Design review of the part built by this model. Coordinates are the model's own, in mm. Face numbers are marked on the shaded views. Coordinates: 2 decimals unless noted, no trailing zeros. Loops run counter-clockwise (first coordinate to the right, second up) from the corner with the lowest first, then second, coordinate; pieces in that order, holes last. Notation, with made-up numbers: (-16.5, 30) -> (8.5, 30) arc R13 cw to (8.5, 43) -> close; hole circle Ø9 at (49, 89). An arc over 180 degrees is marked (long way). Answer as a JSON object with one key per item and string values.
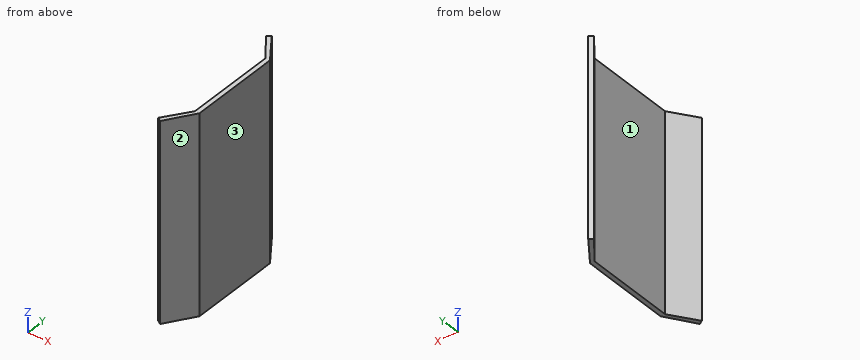
```python
from build123d import *

# Parameters (mm, degrees)
F0_W     = 30
F0_H     = 600
F1_DEPTH = 1300


with BuildPart() as f1:
    # F0 (on Top) → F1 (new body)
    with BuildSketch(Plane.XY):
        with Locations((-14.494546, -122.679873)):
            Rectangle(F0_W, F0_H)
        Polygon((-29.494546, 177.320127), (0.505454, 177.320127), (-124.828876, 354.750561), (-149.332099, 337.441833), align=None)
        Polygon((-119.177751, -603.115286), (0.505454, -422.679873), (-29.494546, -422.679873), (-144.178013, -586.532557), align=None)
    extrude(amount=F1_DEPTH)


solid = f1.part
```
1) Wall thickness on probe 1 along Y at (x, z) = (-102.5, 386.5); probe 2 along X at (y, z) = (-357, 454.5); probe 3 along Y at (x, z) = (-122, 363.5): over which ranges is each line inside the solid? List them lowest first.
Completed:
{"probe 1": "-577.97 to -526.99, 274.87 to 323.14", "probe 2": "-29.49 to 0.51", "probe 3": "-601.24 to -554.85, 300.92 to 350.75"}
2) The part is to be moulded in two halves that separate along Y. For the marked faces 1, 2 and 3, say which applies: pulls with the +Y half, pulls with the -Y half, needs draft (parallel to the pull), parting line crosses it, or undercut.
Completed:
{"face 1": "undercut", "face 2": "pulls with the -Y half", "face 3": "needs draft"}
3) Add section B-B, the plane z = 821.5. Give the boundary of the cut face in (x, y), and give its area (3 significant figures).
Completed:
{"outline": "(-149.33, 337.44) -> (-29.49, 177.32) -> (-29.49, -422.68) -> (-144.18, -586.53) -> (-119.18, -603.12) -> (0.51, -422.68) -> (0.51, 177.32) -> (-124.83, 354.75) -> close", "area": "29,400 mm²"}
4) Add section C-C, the plane y = 123. Give the boundary of the cut face in (x, z), and give its area (3 significant figures).
Completed:
{"outline": "(-29.49, 0) -> (0.51, 0) -> (0.51, 1300) -> (-29.49, 1300) -> close", "area": "39,000 mm²"}
5) Add section A-A, the plane x = -74. Give the boundary of the cut face in (y, z), and give its area (3 significant figures).
Completed:
{"outline": "(-535, 0) -> (-486.27, 0) -> (-486.27, 1300) -> (-535, 1300) -> close; (236.79, 0) -> (282.79, 0) -> (282.79, 1300) -> (236.79, 1300) -> close", "area": "123,000 mm²"}
6) Clearance check with flat-ended pins moving along their axes: pin 1 Ø4 at (x, z) = (-78.5, 905.5) entering from -Y; pin 2 Ø2 at (x, z) = (-129.5, 780) entering from +Y; pin 3 Ø1.5 at (x, z) = (-116.5, 1087) entering from +Y. State where each tip first meets the part, or that it passes through.
Completed:
{"pin 1": "y = -544.8", "pin 2": "y = 352.16", "pin 3": "y = 344.02"}
7) Add section D-D, the plane x = -13. Give the boundary of the cut face in (y, z).
Completed:
{"outline": "(-443.04, 0) -> (196.44, 0) -> (196.44, 1300) -> (-443.04, 1300) -> close"}
